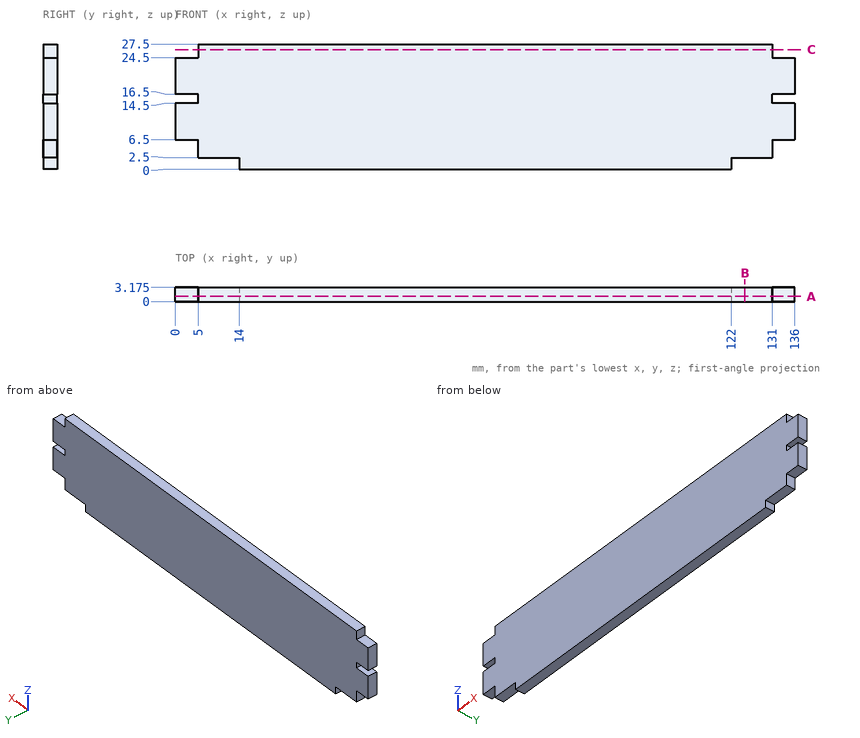
Could you check a few things on this drawing? It's one solid part, dimensions in mm from its lowest x, y, z. Coordinates: 2 decimals unless noted, no trailing zeros. Order: outer loops, then holes, each group sorted by start corner. A loop starts at its lowest first (then second) coordinate and runs counter-clockwise, first axis right, second up. Notation, with made-up numbers: (80.25, 3.25) -> (137.25, 3.25) arc R4 cw to (137.25, 7.25) -> close; hole circle Ø10 at (-31.5, 45.5). An arc over 180 degrees is marked (long way). One line per item, written item: value. Start each with the question number.
1) Imagine slicing it at A-A on y = 1.2. List the corners of the cut face in (x, z) for me, plus the area to 3 significant figures.
2) If I drill on L1, parallel to X at y = 2, z = 3.75; L2, parallel to Z at x = 9, y = 3; L3, parallel to X at y = 1.3, z = 1.75, over which ranges is the centre line in solid material (lowest first)? Write a range as [from, to].
3) I'm going to push flat-ended pins straight in: pin 1 (1.5 mm diameter, centred on y = 1, z = 26, fed in from +X); pin 2 (1 mm diameter, centred on x = 134.5, y = 1.5, fed in from -Z); pin 3 (10 mm diameter, centred on x = 27, z = 14, fed in from -Y); pin 4 (1.6 mm diameter, centred on x = 7.5, y = 1, fed in from -Z). Where does each tip first touch, or does it pass through?
4) Imagine slicing it at B-B on x = 125. List the corners of the cut face in (y, z) for me (3 decimals).
5) Imagine slicing it at C-C on z = 26.25. List the corners of the cut face in (x, y) for me (3 decimals), plus the area to 3 significant figures.
Answer list:
1. outline: (0, 6.5) -> (5, 6.5) -> (5, 2.5) -> (14, 2.5) -> (14, 0) -> (122, 0) -> (122, 2.5) -> (131, 2.5) -> (131, 6.5) -> (136, 6.5) -> (136, 14.5) -> (131, 14.5) -> (131, 16.5) -> (136, 16.5) -> (136, 24.5) -> (131, 24.5) -> (131, 27.5) -> (5, 27.5) -> (5, 24.5) -> (0, 24.5) -> (0, 16.5) -> (5, 16.5) -> (5, 14.5) -> (0, 14.5) -> close
1. area: 3,580 mm2
2. L1: x = [5, 131]
2. L2: z = [2.5, 27.5]
2. L3: x = [14, 122]
3. pin 1: stops at x = 131
3. pin 2: stops at z = 6.5
3. pin 3: stops at y = 0
3. pin 4: stops at z = 2.5
4. outline: (0, 2.5) -> (3.175, 2.5) -> (3.175, 27.5) -> (0, 27.5) -> close
5. outline: (5, 0) -> (131, 0) -> (131, 3.175) -> (5, 3.175) -> close
5. area: 400 mm2
